Verification items for the finished model (mm, model axes). A direction names the side the tool comes from. Give positions to 0.01 mm unless a question says otherwise; leave off trailing zeros. Write each loop counter-clockwise with the first axis right and the second up, starting at its lowest first coordinate (ties: lowest second). Pieces come first, ordered by that corner, then holes. Notation, with made-up numbers: (24.25, 60.5) - (50.25, 60.5) arc R12 ccw to (50.25, 67.5) - close; hole circle Ø4 at (71, 18.25). An arc over 180 degrees is marked (long way). Answer as a JSON object with one key per item and string values. Group by question number.
Item 1: Tool access check on faces 1 (the face through (-54, 48, -5)), 2 (the face through (-54, 62, -5)), 3 (the face through (-58, 55, 4.5)), 4 (the face through (-54.535, 52.253, -19.879)). Record the directions out of +Z, -Z, +X, -X, +Y, -Y that give a thin tool (end or side, any length) a straight path to the whole face; none if there is none.
Item 2: Sectioned sample at D-D, the plane x = -58. Record the boundary of the cut face in (y, z).
Item 3: Sectioned sample at B-B, the plane y = 59.25. Record the boundary of the cut face in (x, z), and give its area (3 significant figures).
Item 4: Scan lines: line 1 along Z through (x, y) = (-55.05, 55); line 2 along Y through (x, z) = (-53.5, 9); line 3 along Y through (x, z) = (-55.25, 5.5). Record each from-to range of solid material in increasing order. Write a range as [from, to].
Item 5: Draft check along Z on faces 5 (the face through (-56.5, 48.5, -19.5)), 6 (the face through (-54.5, 48.5, 14)), 7 (the face through (-61.3, 63.2, -5.7)). Enter one of: +Z half, -Z half, draft (parallel to the pull), parting line (faces both ways), or undercut.
Item 6: Sectioned sample at A-A, the plane y = 55. Record the boundary of the cut face in (x, z), and give its area (3 significant figures).
Item 7: Go/stop test with flat-tipped pins: pin 1 (1 mm diameter, centred on x = -56.5, z = -7.5, fed in from +Y); pin 2 (3 mm diameter, centred on y = 53, z = 2, fed in from -X); pin 3 (0.9 mm diameter, centred on x = -54, z = 1, fed in from -Y). Record where each tip stops, or that it passes through.
Item 8: Sectioned sample at C-C, the plane z = -18. Count the separate pieces of the cut face and the enclosed holes in it, and give its area (3 significant figures).
```python
from build123d import *

# Parameters (mm, degrees)
PAD017_DEPTH    = 9
SKETCH031_W     = 8.5
SKETCH031_H     = 20
PAD018_DEPTH    = 3.5
PAD019_DEPTH    = 7
SKETCH033_R     = 2.75
POCKET013_DEPTH = 5.001
CHAMFER014_SIZE = 1


with BuildPart() as part:
    # Sketch030 → Pad017 (new body, symmetric)
    with BuildSketch(Plane.XZ):
        with BuildLine():
            ThreePointArc((-62.185441, -21.409903), (-57, -5.5), (-62.185441, 10.409903))
            Line((-68.090097, 10.409903), (-62.185441, 10.409903))
            ThreePointArc((-68.090097, -21.409903), (-61.5, -5.5), (-68.090097, 10.409903))
            Line((-68.090097, -21.409903), (-62.185441, -21.409903))
        make_face()
    extrude(amount=PAD017_DEPTH, both=True)

    # Sketch031 → Pad018 (join, symmetric)
    with BuildSketch(Plane.XZ):
        with Locations((-56.25, -5.5)):
            Rectangle(SKETCH031_W, SKETCH031_H)
    extrude(amount=PAD018_DEPTH, both=True)

    # Sketch032 → Pad019 (join, symmetric)
    with BuildSketch(Plane.XZ):
        with BuildLine():
            Line((-52, 14.5), (-57, 14.5))
            Line((-57, 14.5), (-57, 3.624144))
            ThreePointArc((-57, -14.624144), (-55.5, -5.5), (-57, 3.624144))
            Line((-57, -14.624144), (-57, -25.5))
            Line((-57, -25.5), (-52, -25.5))
            Line((-52, -25.5), (-52, 14.5))
        make_face()
    extrude(amount=PAD019_DEPTH, both=True)

    # Sketch033 → Pocket013 (cut, through all)
    with BuildSketch(Plane.YZ.offset(-57)):
        with Locations((0, 9)):
            Circle(SKETCH033_R)
        with Locations((0, -20)):
            Circle(SKETCH033_R)
    extrude(amount=POCKET013_DEPTH, mode=Mode.SUBTRACT)

    # Chamfer014
    chamfer014_edges = [part.edges().sort_by_distance(p)[0] for p in [
        (-57, -7, -20.062072),
        (-54.5, -7, -25.5),
        (-52, -7, -5.5),
        (-54.5, -7, 14.5),
        (-57, -7, 9.062072),
        (-55.5, -7, -5.5),
        (-52, 0, 14.5),
        (-57, 0, 14.5),
        (-54.5, 7, 14.5),
        (-57, 7, -20.062072),
        (-54.5, 7, -25.5),
        (-52, 7, -5.5),
        (-57, 7, 9.062072),
        (-55.5, 7, -5.5),
        (-57, 0, -25.5),
        (-52, 0, -25.5),
        (-68.090097, 0, -21.409903),
        (-68.090097, 0, 10.409903),
        (-61.5, 9, -5.5),
        (-61.5, -9, -5.5),
    ]]
    chamfer(chamfer014_edges, length=CHAMFER014_SIZE)


with BuildPart() as part_1:
    # Body001008 placement: moved
    add(part.part.moved(Location((0, 55, 0))))


solid = part_1.part
```
Geometry check:
{
 "1": {"face 1": "+Z, -Z, +X, -Y", "face 2": "+Z, -Z, +X, +Y", "face 3": "+Z, +Y, -Y", "face 4": "+X"},
 "2": {"outline": "(46, -12.78) - (51.5, -12.78) - (51.5, -15.5) - (58.5, -15.5) - (58.5, -12.78) - (64, -12.78) - (64, 1.78) - (58.5, 1.78) - (58.5, 4.5) - (51.5, 4.5) - (51.5, 1.78) - (46, 1.78) - close"},
 "3": {"outline": "(-67.4, -20.69) - (-67.09, -21.41) - (-62.19, -21.41) arc R27 ccw to (-62.19, 10.41) - (-67.09, 10.41) - (-67.4, 9.69) arc R22.5 cw to start; (-57, -24.5) - (-56, -25.5) - (-53, -25.5) - (-52, -24.5) - (-52, 13.5) - (-53, 14.5) - (-56, 14.5) - (-57, 13.5) - (-57, 3.62) arc R28.5 cw to (-57, -14.62) - close", "area": "335 mm^2"},
 "4": {"line 1": "[-25.5, -22.75], [-17.25, 6.25], [11.75, 14.5]", "line 2": "[48, 52.25], [57.75, 62]", "line 3": "[48, 62]"},
 "5": {"face 5": "draft", "face 6": "+Z half", "face 7": "undercut"},
 "6": {"outline": "(-67.4, -20.69) - (-67.09, -21.41) - (-62.19, -21.41) arc R27 ccw to (-58.92, -15.5) - (-57, -15.5) - (-57, -17.25) - (-52, -17.25) - (-52, 6.25) - (-57, 6.25) - (-57, 4.5) - (-58.92, 4.5) arc R27 ccw to (-62.19, 10.41) - (-67.09, 10.41) - (-67.4, 9.69) arc R22.5 cw to start; (-57, -24.5) - (-56, -25.5) - (-53, -25.5) - (-52, -24.5) - (-52, -22.75) - (-57, -22.75) - close; (-57, 11.75) - (-52, 11.75) - (-52, 13.5) - (-53, 14.5) - (-56, 14.5) - (-57, 13.5) - close", "area": "311 mm^2"},
 "7": {"pin 1": "y = 58.5", "pin 2": "x = -63.38", "pin 3": "y = 48"},
 "8": {"separate pieces": "3", "enclosed holes": "0", "area": "142 mm^2"}
}
